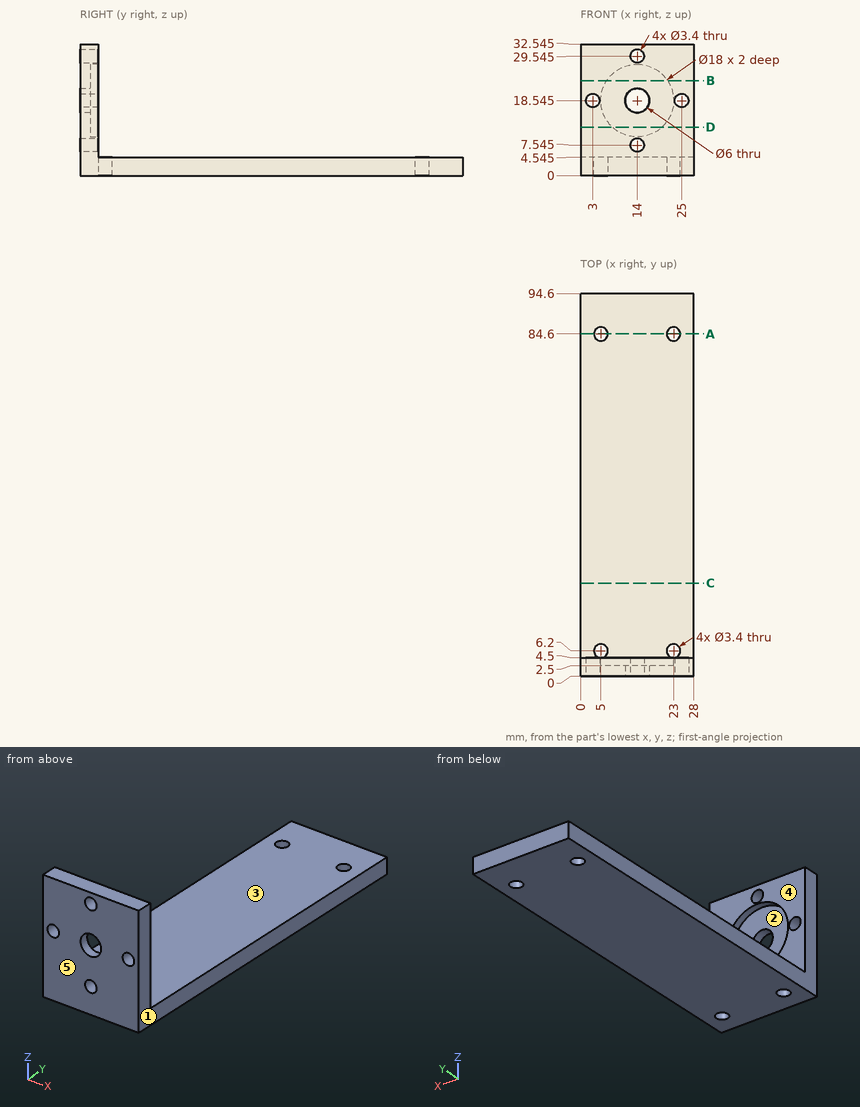
Part print with two shaded views. Sizes in mm from the minimum x, y, z corner. A direction names the side the tool comes from. Round coordinates to 2 decimals unless told otherwise and drop trailing zeros. Write each loop counter-clockwise with the first axis right and the second up, starting at its lowest first coordinate (ties: lowest second). Pieces come first, ordered by that corner, then holes. Notation, with made-up numbers: M -18,48 L -13,48 A23 cw -13,78 Z; hole C 75.5,-39 d8. An arc over 180 degrees is marked long. Answer as CSV lines item,"result". Start each with the question number.
1) Which spindle directions (+Z, -Z, +X, -X, +Y, -Y) get a long thin tool onto all of the face, cutting with end or side? Do the marked faces 4 and 5. Say none if no direction does.
2) Band-saw the part on D-D (z = 12). List the corners of the cut face in (x, y), then the cut area to 3 significant figures.
3) Drill centre lines: L1, parallel to Y at x = 5, z = 2.7; L2, parallel to X at y = 84.6, z = 2.25; L3, parallel to Y at x = 9.5, z = 8. Where is each one in solid material? Low to high.
4) Mould opens along X. For the marked faces 1, 2 and 3 say: +X half, -X half, draft (parallel to the pull), parting line (faces both ways), or undercut.
5) Drop flat-ended pins along their axis: pin 1 (4 mm diameter, centred on x = 14, z = 29.55, fed in from +Y); pin 2 (1 mm diameter, centred on x = 15.5, y = 72.5, fed in from +Z) (3 decimals); pin 3 (10 mm diameter, centred on x = 11.5, z = 18.5, fed in from +Y). Give the stop position or say it passes through.
6) Band-saw the part on A-A (y = 84.6). List the corners of the cut face in (x, z) (3 decimals).
7) Band-saw the part on C-C (y = 23). List the corners of the cut face in (x, z) (3 decimals).
8) Band-saw the part on B-B (z = 23.5). List the corners of the cut face in (x, y).
Worked out:
1,face 4,"+Z, +X, -X, +Y"
1,face 5,"+Z, -Z, +X, -X, -Y"
2,outline,"M 0,0 L 28,0 L 28,4.5 L 20.18,4.5 L 20.18,2.5 L 7.82,2.5 L 7.82,4.5 L 0,4.5 Z"
2,area,"101 mm²"
3,L1,"0 to 4.5, 7.9 to 82.9, 86.3 to 94.6"
3,L2,"0 to 3.3, 6.7 to 21.3, 24.7 to 28"
3,L3,"0 to 4.5"
4,face 1,"+X half"
4,face 2,"undercut"
4,face 3,"draft"
5,pin 1,"y = 4.5"
5,pin 2,"z = 4.545"
5,pin 3,"y = 2.5"
6,outline,"M 0,0 L 3.3,0 L 3.3,4.545 L 0,4.545 Z; M 6.7,0 L 21.3,0 L 21.3,4.545 L 6.7,4.545 Z; M 24.7,0 L 28,0 L 28,4.545 L 24.7,4.545 Z"
7,outline,"M 0,0 L 28,0 L 28,4.545 L 0,4.545 Z"
8,outline,"M 0,0 L 28,0 L 28,4.5 L 21.51,4.5 L 21.51,2.5 L 6.49,2.5 L 6.49,4.5 L 0,4.5 Z"
